Autodesk Inventor part; units mm, degrees
ref_plane "YZ Plane" through (0, 0, 0) normal (1, 0, 0) x (0, 1, 0)
ref_plane "XZ Plane" through (0, 0, 0) normal (0, 1, 0) x (-1, 0, 0)
ref_plane "XY Plane" through (0, 0, 0) normal (0, 0, 1) x (1, 0, 0)
sketch "Sketch1" plane through (0, 0, 0) normal (0, 0, 1) x (1, 0, 0)
  arc A0 (-1, 2.2913) -> (1, 2.2913) centre (0, 0) ccw
  line L0 (33.5703, 31.449) -> (9.177, 7.0557)
  line L1 (31.449, 33.5703) -> (7.0557, 9.177)
  line L2 (-33.5703, 31.449) -> (-9.177, 7.0557)
  line L3 (-31.449, 33.5703) -> (-7.0557, 9.177)
  line L4 (33.5703, -31.449) -> (9.177, -7.0557)
  line L5 (31.449, -33.5703) -> (7.0557, -9.177)
  line L6 (-33.5703, -31.449) -> (-9.177, -7.0557)
  line L7 (-31.449, -33.5703) -> (-7.0557, -9.177)
  arc A1 (-31.449, 33.5703) -> (-33.5703, 31.449) centre (0, 0) ccw
  arc A2 (33.5703, 31.449) -> (31.449, 33.5703) centre (0, 0) ccw
  arc A3 (-33.5703, -31.449) -> (-31.449, -33.5703) centre (0, 0) ccw
  arc A4 (31.449, -33.5703) -> (33.5703, -31.449) centre (0, 0) ccw
  arc A5 (-8.826, 4.7012) -> (-8.826, -4.7012) centre (0, 0) ccw
  arc A6 (-4.7012, -8.826) -> (4.7012, -8.826) centre (0, 0) ccw
  arc A7 (8.826, -4.7012) -> (8.826, 4.7012) centre (0, 0) ccw
  arc A8 (4.7012, 8.826) -> (-4.7012, 8.826) centre (0, 0) ccw
  arc A9 (-8.826, 4.7012) -> (-9.177, 7.0557) centre (-10.5912, 5.6415) ccw
  arc A10 (-9.177, -7.0557) -> (-8.826, -4.7012) centre (-10.5912, -5.6415) ccw
  arc A11 (-4.7012, -8.826) -> (-7.0557, -9.177) centre (-5.6415, -10.5912) ccw
  arc A12 (7.0557, -9.177) -> (4.7012, -8.826) centre (5.6415, -10.5912) ccw
  arc A13 (8.826, -4.7012) -> (9.177, -7.0557) centre (10.5912, -5.6415) ccw
  arc A14 (9.177, 7.0557) -> (8.826, 4.7012) centre (10.5912, 5.6415) ccw
  arc A15 (4.7012, 8.826) -> (7.0557, 9.177) centre (5.6415, 10.5912) ccw
  arc A16 (-7.0557, 9.177) -> (-4.7012, 8.826) centre (-5.6415, 10.5912) ccw
  line L8 (-1, 5.5) -> (1, 5.5)
  line L9 (1, 5.5) -> (1, 2.2913)
  line L10 (-1, 2.2913) -> (-1, 5.5)
  line L11 (-1, 5.5) -> (1, 2.5) construction
  line L12 (1, 5.5) -> (-1, 2.5) construction
  point P0 (8.0517, 5.9304)
  point P1 (5.9304, 8.0517)
  point P2 (-8.0517, 5.9304)
  point P3 (-5.9304, 8.0517)
  point P4 (8.0517, -5.9304)
  point P5 (5.9304, -8.0517)
  point P6 (-8.0517, -5.9304)
  point P7 (-5.9304, -8.0517)
  point P8 (0, 4)
  dimension "d0" = 5
  dimension "d10" = 2
  dimension "d18" = 46
  dimension "d19" = 46
  dimension "d20" = 46
  dimension "d21" = 46
extrude "Extrusion2" add sketch "Sketch1" against normal blind 494
properties part number "propeller"
Verification items for the finished model (mm, model axes). A direction names the side the tool comes from. Round coordinates to 2 decimals unless told otherwise and drop trailing zeros. Write each loop counter-clockwise with the first axis right and the second up, starting at its lowest first coordinate (ties: lowest second). Pieces come first, ordered by that corner, then holes. Notation, with made-up numbers: (53, -29.5) -> (93, -29.5) arc R22 cw to (93, 1.5) -> close; hole circle Ø11 at (43, 85). An arc over 180 degrees is marked (long way). Write each question's results on one line, items separated by ' | '. Start each with the question number.
1. Draft check along Y on faces 1 (the cylindrical face through (0, -10, -244)), 2 (the flat face through (21.54, -19.42, -243.54)), 3 (the flat face through (19.42, 21.54, -243.54)), 4 (the cylindrical face through (10, 0, -244)). Enter one of: +Y half, -Y half, draft (parallel to the pull), parting line (faces both ways), or undercut.
2. Cross-section at C-C (x = -24.5). Enter the section's corners in (y, z).
3. Cross-section at B-B (y = -24). Enter the section's corners in (x, z).
4. Cross-section at A-A (z = -151). Enter the section's corners in (x, y).
5. Depth check by flat-ended pin: P1, Ø1, axis at y = 3.5, z = -319.5, coming from the -X side; P2, Ø3, axis at x = 0, y = 0, coming from the +Z side; P3, Ø1.5, axis at y = -8.5, z = -142, coming from the -X side; P4, Ø2, axis at x = 15.5, z = -215, coming from the +Y side. Enter the tip coordinate at first touch or a pass-through.
6. Set-up check for faces 5 (the flat face through (21.54, 19.42, -243.54)), 6 (the flat face through (-19.42, -21.54, -243.54)), 7 (the flat face through (-21.54, -19.42, -243.54)): record each of +Z, -Z, +X, -X, +Y, -Y from which the full face is reachable in a straight line by a thin tool's end or side.
7. Material ranges on probe 1 along Y at (x, z) = (0, -185); probe 2 along X at (y, z) = (0, -355.5); probe 3 along X at (y, z) = (6, -423.5), recorded low to high. Write a range as from..to.
Solutions:
1) face 1: -Y half | face 2: undercut | face 3: +Y half | face 4: undercut
2) outline: (-26.62, -494) -> (-22.38, -494) -> (-22.38, 0) -> (-26.62, 0) -> close; (22.38, -494) -> (26.62, -494) -> (26.62, 0) -> (22.38, 0) -> close
3) outline: (-26.12, -494) -> (-21.88, -494) -> (-21.88, 0) -> (-26.12, 0) -> close; (21.88, -494) -> (26.12, -494) -> (26.12, 0) -> (21.88, 0) -> close
4) outline: (-33.57, -31.45) arc R46 ccw to (-31.45, -33.57) -> (-7.06, -9.18) arc R2 cw to (-4.7, -8.83) arc R10 ccw to (4.7, -8.83) arc R2 cw to (7.06, -9.18) -> (31.45, -33.57) arc R46 ccw to (33.57, -31.45) -> (9.18, -7.06) arc R2 cw to (8.83, -4.7) arc R10 ccw to (8.83, 4.7) arc R2 cw to (9.18, 7.06) -> (33.57, 31.45) arc R46 ccw to (31.45, 33.57) -> (7.06, 9.18) arc R2 cw to (4.7, 8.83) arc R10 ccw to (-4.7, 8.83) arc R2 cw to (-7.06, 9.18) -> (-31.45, 33.57) arc R46 ccw to (-33.57, 31.45) -> (-9.18, 7.06) arc R2 cw to (-8.83, 4.7) arc R10 ccw to (-8.83, -4.7) arc R2 cw to (-9.18, -7.06) -> close; hole (-1, 2.29) arc R2.5 ccw (long way) to (1, 2.29) -> (1, 5.5) -> (-1, 5.5) -> close
5) P1: stops at x = -9.54 | P2: passes through | P3: stops at x = -11.37 | P4: stops at y = 18.62
6) face 5: +Z, -Z, +X | face 6: +Z, -Z, -Y | face 7: +Z, -Z, -X
7) probe 1: y = -10..-2.5, 5.5..10 | probe 2: x = -10..-2.5, 2.5..10 | probe 3: x = -8.62..8.62
